```python
from build123d import *

# Parameters (mm, degrees)
SKETCH_3_W           = 180
SKETCH_3_H           = 43
EXTRUDE_1_DEPTH      = 12
CUT_EXTRUDE_1_DEPTH  = 52
CUT_EXTRUDE_2_DEPTH  = 5
CUT_EXTRUDE_3_DEPTH  = 5
SKETCH_8_W           = 55
SKETCH_8_H           = 37
CUT_EXTRUDE_4_DEPTH  = 10.5
CUT_EXTRUDE_5_DEPTH  = 5
SKETCH_10_W          = 62.128790526
SKETCH_10_H          = 8.683746703
CUT_EXTRUDE_6_DEPTH  = 8
CUT_EXTRUDE_8_DEPTH  = 9
FILLET_3_R           = 3
FILLET_4_R           = 2.5
SKETCH_12_W          = 15
SKETCH_12_H          = 1.5
CUT_EXTRUDE_9_DEPTH  = 5.5
SKETCH_14_W          = 4.2
SKETCH_14_H          = 4.5
CUT_EXTRUDE_10_DEPTH = 5.5
SKETCH_15_W          = 3
SKETCH_15_H          = 3.5
EXTRUDE_2_DEPTH      = 3


with BuildPart() as part:
    # 草图3 → 凸台-拉伸1 (new body)
    with BuildSketch(Plane(origin=(0, 0, 0), x_dir=(1, 0, 0), z_dir=(0, 1, 0))):
        with Locations((50.068597249, 7.753123643)):
            Rectangle(SKETCH_3_W, SKETCH_3_H)
    extrude(amount=EXTRUDE_1_DEPTH)

    # 草图4 → 切除-拉伸1 (cut)
    with BuildSketch(Plane(origin=(0, 0, 0), x_dir=(1, 0, 0), z_dir=(0, 1, 0))):
        Polygon((-22.469613434, -5.858946979), (26.002261286, -5.858946979), (29.068597249, -13.746876357), (-25.931402751, -13.746876357), align=None)
    extrude(amount=CUT_EXTRUDE_1_DEPTH, mode=Mode.SUBTRACT)

    # 草图5 → 切除-拉伸2 (cut)
    with BuildSketch(Plane(origin=(0, 12, 0), x_dir=(1, 0, 0), z_dir=(0, 1, 0))):
        Polygon((140.068597249, 7.753123643), (140.068597249, 22.753123643), (125.276479966, 22.753123643), (125.276479966, -7.246876357), (140.068597249, -7.246876357), align=None)
    extrude(amount=-CUT_EXTRUDE_2_DEPTH, mode=Mode.SUBTRACT)

    # 草图7 → 切除-拉伸3 (cut)
    with BuildSketch(Plane(origin=(0, 12, 0), x_dir=(1, 0, 0), z_dir=(0, 1, 0))):
        Polygon((125.276479966, 7.753123643), (125.276479966, 25.753123643), (100.500825538, 25.753123643), (100.500825538, -10.246876357), (125.276479966, -10.246876357), align=None)
    extrude(amount=-CUT_EXTRUDE_3_DEPTH, mode=Mode.SUBTRACT)

    # 草图8 → 切除-拉伸4 (cut)
    with BuildSketch(Plane(origin=(0, 12, 0), x_dir=(1, 0, 0), z_dir=(0, 1, 0))):
        with Locations((63.776287419, 7.753123643)):
            Rectangle(SKETCH_8_W, SKETCH_8_H)
    extrude(amount=-CUT_EXTRUDE_4_DEPTH, mode=Mode.SUBTRACT)

    # 草图9 → 切除-拉伸5 (cut)
    with BuildSketch(Plane(origin=(0, 12, 0), x_dir=(1, 0, 0), z_dir=(0, 1, 0))):
        Polygon((91.276287419, 26.253123643), (98.039619719, 26.253123643), (98.039619719, 22.130591531), (98.039619719, 14.279735666), (99.048577369, 12.579380219), (100.500825538, 12.579380219), (100.500825538, 0.629591822), (96.047349228, 0.629591822), (92.132656028, 7.226865659), (92.132656028, 21.255120764), (91.276287419, 21.255120764), align=None)
    extrude(amount=-CUT_EXTRUDE_5_DEPTH, mode=Mode.SUBTRACT)

    # 草图10 → 切除-拉伸6 (cut)
    with BuildSketch(Plane(origin=(0, 12, 0), x_dir=(1, 0, 0), z_dir=(0, 1, 0))):
        with Locations((1.934159822, -6.405003006)):
            Rectangle(SKETCH_10_W, SKETCH_10_H)
    extrude(amount=-CUT_EXTRUDE_6_DEPTH, mode=Mode.SUBTRACT)

    # 草图11 → 切除-拉伸8 (cut)
    with BuildSketch(Plane(origin=(0, 12, 0), x_dir=(1, 0, 0), z_dir=(0, 1, 0))):
        Polygon((32.998555085, -10.746876357), (-36.5396752, -10.746876357), (-36.5396752, 26.253123643), (36.276287419, 26.253123643), (36.276287419, -2.167243749), (32.998555085, -2.063129654), align=None)
    extrude(amount=-CUT_EXTRUDE_8_DEPTH, mode=Mode.SUBTRACT)

    # 圆角3
    fillet_3_edges = [part.edges().sort_by_distance(p)[0] for p in [
        (-39.931402751, 6, -29.253123643),
        (140.068597249, 6, -29.253123643),
        (140.068597249, 6, 13.746876357),
        (-39.931402751, 6, 13.746876357),
    ]]
    fillet(fillet_3_edges, radius=FILLET_3_R)

    # 圆角4
    fillet_4_edges = [part.edges().sort_by_distance(p)[0] for p in [
        (83.068597249, 0, 13.746876357),
        (50.068597249, 0, -29.253123643),
        (-31.431402751, 0, 13.746876357),
        (-39.931402751, 0, -7.753123643),
        (140.068597249, 0, -7.753123643),
        (-39.052723094, 0, -28.374443987),
        (-39.052723094, 0, 12.8681967),
        (139.189917593, 0, 12.8681967),
        (139.189917593, 0, -28.374443987),
    ]]
    fillet(fillet_4_edges, radius=FILLET_4_R)

    # 草图12 → 切除-拉伸9 (cut)
    with BuildSketch(Plane(origin=(0, 12, 0), x_dir=(1, 0, 0), z_dir=(0, 1, 0))):
        with Locations((28.776287419, 27.003123643)):
            Rectangle(SKETCH_12_W, SKETCH_12_H)
    extrude(amount=-CUT_EXTRUDE_9_DEPTH, mode=Mode.SUBTRACT)

    # 草图14 → 切除-拉伸10 (cut)
    with BuildSketch(Plane(origin=(-36.5396752, 0, 0), x_dir=(0, 0, -1), z_dir=(1, 0, 0))):
        with Locations((13.253123643, 6.7)):
            Rectangle(SKETCH_14_W, SKETCH_14_H)
    extrude(amount=-CUT_EXTRUDE_10_DEPTH, mode=Mode.SUBTRACT)

    # 草图15 → 凸台-拉伸2 (add)
    with BuildSketch(Plane(origin=(0, 3, 0), x_dir=(1, 0, 0), z_dir=(0, 1, 0))):
        with Locations((-28.0396752, 13.253123643)):
            Rectangle(SKETCH_15_W, SKETCH_15_H)
    extrude(amount=EXTRUDE_2_DEPTH)


with BuildPart() as body_2:
    # 镜向3: mirrored copy
    add(part.part.mirror(Plane(origin=(0, 0, -39.253123643), x_dir=(1, 0, 0), z_dir=(0, 0, -1))))


solid = body_2.part
```
Source: CAD feature listing. Evaluate the final solid. Frame: model axes, mm. A direction names the side the tool comes from. Round coordinates to 2 decimals unless told otherwise and drop trailing zeros. Loops run counter-clockwise (first coordinate to the right, second up) from the corner with the lowest first, then second, coordinate; pieces in that order, holes last.
1. Section query A-A on z = -61.5. Output: boundary loops of the cut face in (x, y), and give its area (3 significant figures).
2. Mould query, pull axis X, two halves, no side actions, for faces 5 (the flat face through (140.069, 5, -71)), 6 (the flat face through (133, 10, -55.753)), 7 (the flat face through (-29.54, 4, -65)). Classes: released by +X, released by -X, zero draft, split by the parting line, or undercut.
3. Ray query, L1, parallel to X at y = 11, z = -84.5; L2, parallel to X at y = 11.75, z = -87; L3, parallel to X at y = 5.5, z = -86.5. Return the intervals inside material, ascending.
4. Section query C-C on x = 4.5. Output: boundary loops of the cut face in (y, z), and give its area (3 significant figures).
5. Section query D-D on z = -75.5. Output: boundary loops of the cut face in (x, y).
6. Section query B-B on x = 113. Output: boundary loops of the cut face in (y, z).
7. Contact query for flat-ended pins moving along their axis: pin 1 (1.5 mm diameter, centred on y = 8.5, z = -81.5, fed in from +X); pin 2 (2.5 mm diameter, centred on x = 12, y = 1, fed in from -Z); pin 3 (5 mm diameter, centred on x = 3.5, y = 7.5, fed in from -Z). Output: stop coordinate, or through.
8. Access query for faces 1 (the flat face through (49, 0, -70)), 2 (the flat face through (-38, 7, -63.153)), 3 (the flat face through (113, 10, -88.753)), 4 (the flat face through (1, 1, -84.365)). Directions: +Z, -Z, +X, -X, +Y, -Y. A direction counts if a zero-diameter tool reaches every point of the face in a straight line with its end or side. Return the directions, or none.
Answers below:
1. outline: (-39.93, 2.5) arc R2.5 ccw to (-37.43, 0) - (137.57, 0) arc R2.5 ccw to (140.07, 2.5) - (140.07, 7) - (100.5, 7) - (100.5, 12) - (98.04, 12) - (98.04, 7) - (92.13, 7) - (92.13, 12) - (91.28, 12) - (91.28, 1.5) - (36.28, 1.5) - (36.28, 3) - (-36.54, 3) - (-36.54, 12) - (-39.93, 12) - close
1. area: 697 mm2
2. face 5: released by +X
2. face 6: zero draft
2. face 7: undercut
3. L1: x = -39.93 to -36.54, 33 to 36.28, 91.28 to 100.5
3. L2: x = -39.93 to -36.54, 33 to 36.28, 91.28 to 100.5, 125.28 to 140.07
3. L3: x = -39.93 to -36.54, 33 to 36.28, 91.28 to 140.07
4. outline: (0, -84.37) - (3, -84.37) - (3, -52.25) - (12, -52.25) - (12, -49.25) - (2.5, -49.25) arc R2.5 ccw to (0, -51.75) - close
4. area: 131 mm2
5. outline: (-39.93, 2.5) arc R2.5 ccw to (-37.43, 0) - (137.57, 0) arc R2.5 ccw to (140.07, 2.5) - (140.07, 7) - (94.64, 7) - (94.64, 12) - (91.28, 12) - (91.28, 1.5) - (36.28, 1.5) - (36.28, 3) - (-36.54, 3) - (-36.54, 12) - (-39.93, 12) - close
6. outline: (0, -89.75) arc R2.5 ccw to (2.5, -92.25) - (12, -92.25) - (12, -88.75) - (7, -88.75) - (7, -52.75) - (12, -52.75) - (12, -49.25) - (2.5, -49.25) arc R2.5 ccw to (0, -51.75) - close
7. pin 1: stops at x = 100.5
7. pin 2: stops at z = -84.37
7. pin 3: stops at z = -52.25
8. face 1: +Z, -Z, +X, -X, -Y
8. face 2: -X
8. face 3: +Y
8. face 4: -Z, +Y, -Y
